Build history of the part. All positions in model axes, mm. A direction names the side the tool comes from. Coordinates: 2 decimals unless noted, no trailing zeros. Loops run counter-clockwise (first coordinate to the right, second up) from the corner with the lowest first, then second, coordinate; pieces in that order, holes last.
(1) Tool access for faces 1 (the face through (1.27, 2.6, 2.9)), 2 (the face through (0.72, 1.77, -0.69)), 3 (the face through (3, -2, -0.94)), 4 (the face through (-3.416, -1.9, -0.5)), 5 (the face through (0, 2, 2.73)): list every direction of +Z, -Z, +X, -X, +Y, -Y with a clear straight run to the whole face (end or side of a thin tool).
(2) Slice it at B-B (y = 1.75). Give the number of separate pieces and of enclosed holes in the cut face, and give its area (3 significant figures).
(3) Wall check: L1, parallel to Z at x = 6, y = 1.75; L2, parallel to X at y = -1, z = -0.75; L3, parallel to Y at x = -2, z = 1.75. Give the ranges that are in metal, low to high.
(4) Flat gauge pins, fed straight in: P1, Ø1.4, axis at x = -3, y = -1, coming from the -Z side; P2, Ø1.1, axis at y = 2.5, z = 2.5, coming from the +X side (3 decimals); P3, Ø1.1, axis at x = 0, y = -2, coming from the +Z side. Where does each tip first touch, or does it go through?
(5) Two-plate mould, pull along Z, no slides. Class faces 6 (the face through (0, 0, -1)), 7 (the face through (0.73, 1.77, 0.66)), 8 (the face through (0, 1, 3.238)): pulls with the +Z half, pulls with the -Z half, needs draft (parallel to the pull), parting line crosses it, or undercut.
(6) Slice it at A-A (z = 2.5). Give the cut face in (x, y) (3 decimals), and give its area (3 significant figures).
(7) Slice it at D-D (y = -3). Give the cut face in (x, z).
(8) Slice it at C-C (z = 1.75). Give the cut face in (x, y) (3 decimals).
from build123d import *

# Parameters (mm, degrees)
SKETCH1_W           = 13.97
SKETCH1_H           = 6.477
BOSS_EXTRUDE1_DEPTH = 1.524
SKETCH2_W           = 2.54
SKETCH2_H           = 0.508
BOSS_EXTRUDE2_DEPTH = 1.016
SKETCH3_W           = 2.54
SKETCH3_H           = 1.016
BOSS_EXTRUDE3_DEPTH = 0.508
BOSS_EXTRUDE4_DEPTH = 0.508
SKETCH5_W           = 1.195099264
SKETCH5_H           = 0.512185399
BOSS_EXTRUDE5_DEPTH = 0.508
BOSS_EXTRUDE6_DEPTH = 3.81


with BuildPart() as part:
    # Sketch1 → Boss-Extrude1 (new body)
    with BuildSketch(Plane(origin=(0, 0, 0), x_dir=(1, 0, 0), z_dir=(0, 1, 0))):
        Rectangle(SKETCH1_W, SKETCH1_H)
    extrude(amount=BOSS_EXTRUDE1_DEPTH)

    # Sketch2 → Boss-Extrude2 (add)
    with BuildSketch(Plane(origin=(0, 1.524, 0), x_dir=(1, 0, 0), z_dir=(0, 1, 0))):
        with Locations((0, -2.9845)):
            Rectangle(SKETCH2_W, SKETCH2_H)
    extrude(amount=BOSS_EXTRUDE2_DEPTH)

    # Sketch3 → Boss-Extrude3 (add)
    with BuildSketch(Plane(origin=(0, 2.54, 0), x_dir=(1, 0, 0), z_dir=(0, 1, 0))):
        with Locations((0, -2.7305)):
            Rectangle(SKETCH3_W, SKETCH3_H)
    extrude(amount=BOSS_EXTRUDE3_DEPTH)

    # Sketch4 → Boss-Extrude4 (add)
    with BuildSketch(Plane(origin=(0, 1.524, 0), x_dir=(1, 0, 0), z_dir=(0, 1, 0))):
        Polygon((-6.477, -2.7305), (-6.477, 2.7305), (6.477, 2.7305), (6.477, -2.7305), (1.27, -2.7305), (1.27, -3.2385), (6.985, -3.2385), (6.985, 3.2385), (-6.985, 3.2385), (-6.985, -3.2385), (-1.27, -3.2385), (-1.27, -2.7305), align=None)
    extrude(amount=BOSS_EXTRUDE4_DEPTH)

    # Sketch5 → Boss-Extrude5 (add)
    with BuildSketch(Plane(origin=(0, 1.524, 0), x_dir=(1, 0, 0), z_dir=(0, 1, 0))):
        Polygon((-1.643378995, -1.3589), (-2.32629286, -1.3589), (-2.32629286, 0.435883001), (-2.802198459, -0.710131829), (-3.250360683, -0.710131829), (-3.726266283, 0.435883001), (-3.726266283, -1.3589), (-4.375034454, -1.3589), (-4.375034454, 1.338609766), (-3.587549404, 1.338609766), (-3.007606145, 0.016531206), (-2.429796993, 1.338609766), (-1.643378995, 1.338609766), align=None)
        Polygon((1.190713543, -1.3589), (0.410697863, -1.3589), (-0.119093908, -0.495120666), (-0.659022682, -1.3589), (-1.404359143, -1.3589), (-0.488294216, 0.002125991), (-1.370213449, 1.338609766), (-0.590731296, 1.338609766), (-0.094551691, 0.525515445), (0.41123139, 1.338609766), (1.15656785, 1.338609766), (0.274648617, 0.028802314), align=None)
        with Locations((1.958991641, -0.180873583)):
            Rectangle(SKETCH5_W, SKETCH5_H)
        with BuildLine():
            add(Edge.make_bspline(
                [(4.946739799, -0.455106182), (4.94605947, -0.489662616), (4.944721084, -0.557644192), (4.929944432, -0.657573198), (4.908066939, -0.753857587), (4.87622275, -0.845773262), (4.83676263, -0.933299855), (4.786314976, -1.014033908), (4.728286007, -1.089798027), (4.682686747, -1.134274984), (4.659702565, -1.156693473)],
                knots=[0, 0, 0, 0, 0.000103592, 0.000203793, 0.000302407, 0.000399423, 0.000495152, 0.000589768, 0.000684431, 0.000780639, 0.000780639, 0.000780639, 0.000780639], degree=3))
            add(Edge.make_bspline(
                [(4.659702565, -1.156693473), (4.635406854, -1.177518935), (4.586634173, -1.219325227), (4.505001964, -1.272541327), (4.417255575, -1.319210004), (4.321943242, -1.358475376), (4.21766177, -1.389721666), (4.102769549, -1.411786565), (3.976570704, -1.42510693), (3.888613592, -1.426478259), (3.84287356, -1.427191386)],
                knots=[0, 0, 0, 0, 9.5912e-05, 0.000192539, 0.000291587, 0.000393737, 0.000501257, 0.00061761, 0.000744227, 0.000881409, 0.000881409, 0.000881409, 0.000881409], degree=3))
            add(Edge.make_bspline(
                [(3.84287356, -1.427191386), (3.794477078, -1.426480894), (3.700952929, -1.425107899), (3.566044943, -1.41446127), (3.441363909, -1.399893023), (3.327411732, -1.377455404), (3.223622789, -1.351832076), (3.129158438, -1.324471539), (3.044025447, -1.296336264), (2.991260446, -1.274703465), (2.966289592, -1.264465817)],
                knots=[0, 0, 0, 0, 0.000145167, 0.00028053, 0.0004058, 0.000521528, 0.000628671, 0.000726434, 0.000816529, 0.000897473, 0.000897473, 0.000897473, 0.000897473], degree=3))
            Line((2.966289592, -1.264465817), (2.966289592, -0.675986135))
            Line((2.966289592, -0.675986135), (3.028178661, -0.675986135))
            add(Edge.make_bspline(
                [(3.028178661, -0.675986135), (3.0461748, -0.686599796), (3.084373728, -0.709128543), (3.133224942, -0.739286447), (3.177777625, -0.764600081), (3.217135707, -0.784178099), (3.261692934, -0.803718246), (3.292967822, -0.816879929), (3.309347103, -0.823772964)],
                knots=[0, 0, 0, 0, 6.2677e-05, 0.00013304, 0.000172217, 0.000216358, 0.000264842, 0.000318154, 0.000318154, 0.000318154, 0.000318154], degree=3))
            add(Edge.make_bspline(
                [(3.309347103, -0.823772964), (3.34138122, -0.83629162), (3.405232789, -0.861244261), (3.487688702, -0.886196407), (3.555852103, -0.901383164), (3.609882629, -0.909220124), (3.666539884, -0.91414204), (3.705213193, -0.91471392), (3.724964213, -0.915005988)],
                knots=[0, 0, 0, 0, 0.000103158, 0.000205619, 0.000258049, 0.000312526, 0.000369283, 0.000428526, 0.000428526, 0.000428526, 0.000428526], degree=3))
            add(Edge.make_bspline(
                [(3.724964213, -0.915005988), (3.742755847, -0.914663026), (3.779288763, -0.913958795), (3.835093925, -0.909188759), (3.892833649, -0.900129367), (3.951474932, -0.889677579), (4.008759587, -0.875016308), (4.060932423, -0.853514292), (4.107961529, -0.827647814), (4.134493655, -0.805366147), (4.147517167, -0.794429009)],
                knots=[0, 0, 0, 0, 5.3377e-05, 0.000109602, 0.000167852, 0.000228648, 0.00028831, 0.000344784, 0.000397592, 0.000448504, 0.000448504, 0.000448504, 0.000448504], degree=3))
            add(Edge.make_bspline(
                [(4.147517167, -0.794429009), (4.164388109, -0.775955433), (4.197780925, -0.73939051), (4.229692696, -0.685066402), (4.247298267, -0.63645426), (4.257736249, -0.594516462), (4.262394262, -0.546619491), (4.263331382, -0.512910261), (4.263825935, -0.495120666)],
                knots=[0, 0, 0, 0, 7.4941e-05, 0.000148331, 0.000186985, 0.000229817, 0.0002776, 0.000330995, 0.000330995, 0.000330995, 0.000330995], degree=3))
            add(Edge.make_bspline(
                [(4.263825935, -0.495120666), (4.263214375, -0.480167371), (4.262020954, -0.450986903), (4.255637945, -0.408563008), (4.242263097, -0.36988429), (4.225355871, -0.334193666), (4.203453064, -0.30241436), (4.179789927, -0.272527925), (4.151721285, -0.246927559), (4.131136036, -0.232414579), (4.120840844, -0.225156279)],
                knots=[0, 0, 0, 0, 4.4896e-05, 8.7611e-05, 0.000128103, 0.000167236, 0.000205709, 0.000243623, 0.00028138, 0.000319155, 0.000319155, 0.000319155, 0.000319155], degree=3))
            add(Edge.make_bspline(
                [(4.120840844, -0.225156279), (4.104707777, -0.21545969), (4.071734836, -0.195641694), (4.016892486, -0.17391933), (3.957698389, -0.156300514), (3.895021078, -0.146296935), (3.832643779, -0.139181726), (3.773581815, -0.133780992), (3.718958649, -0.130345567), (3.684064997, -0.12987875), (3.667343356, -0.129655044)],
                knots=[0, 0, 0, 0, 5.6382e-05, 0.000115235, 0.000176356, 0.000241352, 0.000305279, 0.000364741, 0.000419255, 0.000469417, 0.000469417, 0.000469417, 0.000469417], degree=3))
            add(Edge.make_bspline(
                [(3.667343356, -0.129655044), (3.617843369, -0.130527073), (3.519806509, -0.132254165), (3.39941227, -0.147583805), (3.307040027, -0.161526065), (3.242965144, -0.173689398), (3.18341676, -0.184924031), (3.145528801, -0.193734262), (3.127414582, -0.19794643)],
                knots=[0, 0, 0, 0, 0.000148416, 0.000293945, 0.000363592, 0.000428682, 0.000489579, 0.000545365, 0.000545365, 0.000545365, 0.000545365], degree=3))
            Line((3.127414582, -0.19794643), (3.068726671, -0.19794643))
            Line((3.068726671, -0.19794643), (3.068726671, 1.338609766))
            Line((3.068726671, 1.338609766), (4.878448413, 1.338609766))
            Line((4.878448413, 1.338609766), (4.878448413, 0.826424367))
            Line((4.878448413, 0.826424367), (3.717494843, 0.826424367))
            Line((3.717494843, 0.826424367), (3.717494843, 0.373460405))
            add(Edge.make_bspline(
                [(3.717494843, 0.373460405), (3.737585525, 0.374808914), (3.780939543, 0.377718884), (3.836285807, 0.379582643), (3.882002433, 0.380815422), (3.913647804, 0.38204891), (3.941040243, 0.382621495), (3.957937284, 0.382558752), (3.965584645, 0.382530355)],
                knots=[0, 0, 0, 0, 6.0404e-05, 0.000130347, 0.000166109, 0.000197605, 0.000225354, 0.000248295, 0.000248295, 0.000248295, 0.000248295], degree=3))
            add(Edge.make_bspline(
                [(3.965584645, 0.382530355), (3.997606389, 0.381939784), (4.060302129, 0.380783498), (4.152627332, 0.374010631), (4.24113585, 0.361615555), (4.326092456, 0.344887486), (4.40663311, 0.322371742), (4.482865869, 0.295381841), (4.554235733, 0.262433225), (4.598396472, 0.235689641), (4.620221608, 0.222472418)],
                knots=[0, 0, 0, 0, 9.6072e-05, 0.0001881, 0.000277512, 0.000364043, 0.000447664, 0.000528163, 0.000606453, 0.000682954, 0.000682954, 0.000682954, 0.000682954], degree=3))
            add(Edge.make_bspline(
                [(4.620221608, 0.222472418), (4.64515183, 0.205211361), (4.6948374, 0.170810326), (4.759231976, 0.10669888), (4.816173661, 0.035295495), (4.863168477, -0.045457051), (4.900760282, -0.134880977), (4.928000594, -0.233413985), (4.943911899, -0.341302226), (4.945775058, -0.416281835), (4.946739799, -0.455106182)],
                knots=[0, 0, 0, 0, 9.0809e-05, 0.000180982, 0.000271389, 0.000364173, 0.000460291, 0.000561647, 0.000670074, 0.000786505, 0.000786505, 0.000786505, 0.000786505], degree=3))
        make_face()
    extrude(amount=BOSS_EXTRUDE5_DEPTH)

    # Sketch6 → Boss-Extrude6 (add)
    with BuildSketch(Plane.XZ):
        Polygon((-3.4163, 0), (-2.413, 0.9398), (2.413, 0.9398), (3.4163, 0), (3.4163, -0.9398), (2.159, -0.9398), (2.159, -0.0762), (-2.159, -0.0762), (-2.159, -0.9398), (-3.4163, -0.9398), align=None)
    extrude(amount=BOSS_EXTRUDE6_DEPTH)


solid = part.part
Response values:
1. face 1: +Z, -Z, +X, +Y
1. face 2: +Y
1. face 3: -Z, +X, -X, -Y
1. face 4: +Z, -Z, -X, -Y
1. face 5: none
2. separate pieces: 5
2. enclosed holes: 1
2. area: 32.6 mm2
3. L1: z = -3.24 to -2.73, 2.73 to 3.24
3. L2: x = -3.42 to -2.16, 2.16 to 3.42
3. L3: y = 0 to 1.52
4. P1: stops at z = -0.94
4. P2: stops at x = 6.985
4. P3: stops at z = 0.94
5. face 6: needs draft
5. face 7: undercut
5. face 8: pulls with the +Z half
6. outline: (-6.985, 0) - (6.985, 0) - (6.985, 2.032) - (6.477, 2.032) - (6.477, 1.524) - (-6.477, 1.524) - (-6.477, 2.032) - (-6.985, 2.032) - close; (-1.27, 2.54) - (1.27, 2.54) - (1.27, 3.048) - (-1.27, 3.048) - close
6. area: 23.1 mm2
7. outline: (-3.42, -0.94) - (-2.16, -0.94) - (-2.16, -0.08) - (2.16, -0.08) - (2.16, -0.94) - (3.42, -0.94) - (3.42, 0) - (2.41, 0.94) - (-2.41, 0.94) - (-3.42, 0) - close
8. outline: (-6.985, 0) - (6.985, 0) - (6.985, 2.032) - (6.477, 2.032) - (6.477, 1.524) - (-6.477, 1.524) - (-6.477, 2.032) - (-6.985, 2.032) - close
